from build123d import *

# Parameters (mm, degrees)
F1_DEPTH    = 80
F2_R        = 5
F3_T1_DEPTH = 105.4
F4_T1_DEPTH = 105.4
F5_R        = 5.08


# Not quite as in the source:
# - a fillet or chamfer that OpenCascade refuses, or shapes differently, is made with other operations: its cross-section is extruded or revolved along the edge and cut away or added


with BuildPart() as f1:
    # F0 (on Right) → F1 (new body)
    with BuildSketch(Plane.YZ):
        Polygon((-65.3676100316, -25.1990987622), (-71.8711540103, -44.1121608019), (-61.2964517447, -44.1121608019), (-55.9110790118, -28.4508707515), align=None)
        Polygon((-61.2964517447, -44.1121608019), (-71.8711540103, -44.1121608019), (-71.8711540103, -67.0164749026), (18.1288459897, -67.0164749026), (18.1288459897, -44.1121608019), (-36.4091803752, -44.1121608019), (-47.0806523531, -44.1121608019), (-47.2488089486, -44.1121608019), align=None)
        Polygon((-47.220791987, -44.0451827606), (-47.2488089486, -44.1121608019), (-47.0806523531, -44.1121608019), align=None)
        Polygon((-47.2488089486, -44.031792393), (-47.2488089486, -44.1121608019), (-47.220791987, -44.0451827606), align=None)
        Polygon((-47.220791987, -44.0451827606), (-47.0806523531, -44.1121608019), (-36.4091803752, -44.1121608019), (-3.2924475957, 35.0575196106), (-12.5178559501, 38.9165143882), align=None)
    extrude(amount=F1_DEPTH)

    # F2
    f2_edges = [f1.edges().sort_by_distance(p)[0] for p in [
        (40, -71.871154, -44.112161),
    ]]
    fillet(f2_edges, radius=F2_R)

    # F3: fillet of radius 5.08 on 2 edges, made by hand

    # F3_s2 → F3_t1 (cut)
    with BuildSketch(Plane.YZ.offset(-12.7)):
        with BuildLine():
            ThreePointArc((-5.2528169427, 30.3710121665), (-5.2392727341, 34.2590522484), (-7.9789550397, 37.0178889576))
            Line((-7.9789550397, 37.0178889576), (-3.2924475957, 35.0575196106))
            Line((-3.2924475957, 35.0575196106), (-5.2528169427, 30.3710121665))
        make_face()
        with BuildLine():
            ThreePointArc((-14.4782252971, 34.2300069441), (-11.719388588, 36.9696892498), (-7.8313485061, 36.9561450412))
            Line((-7.8313485061, 36.9561450412), (-12.5178559501, 38.9165143882))
            Line((-12.5178559501, 38.9165143882), (-14.4782252971, 34.2300069441))
        make_face()
    extrude(amount=F3_T1_DEPTH, mode=Mode.SUBTRACT)

    # F4: fillet of radius 5.08 on 2 edges, made by hand

    # F4_s2 → F4_t1 (cut)
    with BuildSketch(Plane.YZ.offset(-12.7)):
        with BuildLine():
            ThreePointArc((-60.7149967698, -26.798970581), (-57.801944305, -29.3740753285), (-57.5629791823, -33.2547885096))
            Line((-57.5629791823, -33.2547885096), (-55.9110790118, -28.4508707515))
            Line((-55.9110790118, -28.4508707515), (-60.7149967698, -26.798970581))
        make_face()
        with BuildLine():
            ThreePointArc((-67.0195102022, -30.0030165203), (-64.4444054547, -27.0899640554), (-60.5636922735, -26.8509989328))
            Line((-60.5636922735, -26.8509989328), (-65.3676100316, -25.1990987622))
            Line((-65.3676100316, -25.1990987622), (-67.0195102022, -30.0030165203))
        make_face()
    extrude(amount=F4_T1_DEPTH, mode=Mode.SUBTRACT)

    # F5
    f5_edges = [f1.edges().sort_by_distance(p)[0] for p in [
        (40, -36.40918, -44.112161),
    ]]
    fillet(f5_edges, radius=F5_R)


solid = f1.part
Check sheet for the modelled part. Datum: model origin and axes. Units: mm. A direction names the side the tool comes from. Coordinates: 2 decimals unless noted, no trailing zeros. Write each loop counter-clockwise with the first axis right and the second up, starting at its lowest first coordinate (ties: lowest second). Pieces come first, ordered by that corner, then holes.
Item 1: Access from +Z, -Z, +X, -X, +Y, -Y to the whole of each face (thin tool, end or side, straight path). Record for faces 4 (the face through (39, -54, -44.112)), 5 (the face through (39.44, -30.62, -4.36)), 6 (the face through (39, -71.871, -56)), 7 (the face through (39, -5, -44.112)).
Numbers:
face 4: +X, -X
face 5: +Z, +X, -X
face 6: +Z, -Z, +X, -X, -Y
face 7: +X, -X, +Y
Item 2: Cross-section at C-C on y = -22. Record the boundary of the cut face in (x, z), then the cut area to 3 significant figures.
Numbers:
outline: (0, -67.02) - (80, -67.02) - (80, -44.11) - (0, -44.11) - close; (0, -9.67) - (80, -9.67) - (80, 16.25) - (0, 16.25) - close
area: 3,910 mm2
Item 3: Depth check by flat-ended pin: pin 1 Ø4 at (x, y) = (44, -51.5) entering from +Z; pin 2 Ø10 at (x, z) = (25, 26.5) entering from -Y; pin 3 Ø4 at (x, z) = (59.5, -24) entering from +Y. Enter the tip coordinate at first touch or a pass-through.
Numbers:
pin 1: stops at z = -44.11
pin 2: stops at y = -19.8
pin 3: stops at y = -27.16
Item 4: Cross-section at D-D on y = -52. Record the boundary of the cut face in (x, z), then the cut area to 3 significant figures.
Numbers:
outline: (0, -67.02) - (80, -67.02) - (80, -44.11) - (0, -44.11) - close
area: 1,830 mm2
Item 5: Mould release check, pull along Z, two halves, no side actions. Record for faces 1 (the face through (39.44, -69.277, -36.569)), 2 (the face through (39.44, -59.456, -38.759)), 3 (the face through (39, 18.129, -56)): released by +Z, released by -Z, zero draft, split by the parting line, or undercut.
Numbers:
face 1: released by +Z
face 2: undercut
face 3: zero draft
Item 6: Cross-section at B-B on z = -35.5. Record the boundary of the cut face in (x, y), then the cut area to 3 significant figures.
Numbers:
outline: (0, -68.91) - (80, -68.91) - (80, -58.34) - (0, -58.34) - close; (0, -43.65) - (80, -43.65) - (80, -32.81) - (0, -32.81) - close
area: 1,710 mm2
Item 7: Scan lines: probe 1 along Z at (x, y) = (33, -1); probe 2 along Z at (x, y) = (38, -11.5); probe 3 along Y at (x, z) = (53.5, -23). Record each from-to range of solid material in increasing order.
Numbers:
probe 1: z = -67.02 to -44.11
probe 2: z = -67.02 to -44.11, 15.44 to 37.05
probe 3: y = -38.42 to -27.58
